```python
from build123d import *

# Parameters (mm, degrees)
SKETCH2_R                       = 11.10996
BOSS_EXTRUDE1_DEPTH             = 4.7625
SKETCH3_W                       = 3.175
SKETCH3_H                       = 181.991160274
CUT_EXTRUDE1_DEPTH              = 0.396875
FILLET1_R                       = 0.79375
F_9_64_0_14063_DIAMETER_HOLE1_D = 3.572002


with BuildPart() as part:
    # Sketch2 → Boss-Extrude1 (new body)
    with BuildSketch(Plane(origin=(0, 0, 0), x_dir=(0, 0, -1), z_dir=(1, 0, 0))):
        with BuildLine():
            Line((81.02619141, 88.258519733), (35.921024484, 114.3))
            ThreePointArc((35.921024484, 114.3), (0, 63.5), (-35.921024484, 114.3))
            Line((-35.921024484, 114.3), (-81.02619141, 88.258519733))
            ThreePointArc((-81.02619141, 88.258519733), (-54.99261314, 31.75), (-116.947215895, 26.041480267))
            Line((-116.947215895, 26.041480267), (-116.947215895, -26.041480267))
            ThreePointArc((-116.947215895, -26.041480267), (-54.99261314, -31.75), (-81.02619141, -88.258519733))
            Line((-81.02619141, -88.258519733), (-35.921024484, -114.3))
            ThreePointArc((-35.921024484, -114.3), (0, -63.5), (35.921024484, -114.3))
            Line((35.921024484, -114.3), (81.02619141, -88.258519733))
            ThreePointArc((81.02619141, -88.258519733), (54.99261314, -31.75), (116.947215895, -26.041480267))
            Line((116.947215895, -26.041480267), (116.947215895, 26.041480267))
            ThreePointArc((116.947215895, 26.041480267), (54.99261314, 31.75), (81.02619141, 88.258519733))
        make_face()
        with Locations(Location((0, 0, 0), (0, 0, 180))):
            Circle(SKETCH2_R, mode=Mode.SUBTRACT)
    extrude(amount=BOSS_EXTRUDE1_DEPTH)

    # Sketch3 → Cut-Extrude1 (cut)
    with BuildSketch(Plane.ZY):
        with Locations((0, 101.6)):
            Rectangle(SKETCH3_W, SKETCH3_H)
        Polygon((167.586415056, 94.92297474), (165.998915056, 97.672605397), (8.389946993, 6.67702526), (9.977446993, 3.927394603), align=None)
        Polygon((165.998915056, -97.672605397), (167.586415056, -94.92297474), (9.977446993, -3.927394603), (8.389946993, -6.67702526), align=None)
        with Locations((0, -101.6)):
            Rectangle(SKETCH3_W, SKETCH3_H)
        Polygon((-167.586415056, -94.92297474), (-165.998915056, -97.672605397), (-8.389946993, -6.67702526), (-9.977446993, -3.927394603), align=None)
        Polygon((-165.998915056, 97.672605397), (-167.586415056, 94.92297474), (-9.977446993, 3.927394603), (-8.389946993, 6.67702526), align=None)
    extrude(amount=-CUT_EXTRUDE1_DEPTH, mode=Mode.SUBTRACT)

    # Fillet1
    fillet1_edges = [part.edges().sort_by_distance(p)[0] for p in [
        (2.38125, 88.258519733, 81.02619141),
        (2.38125, 114.3, 35.921024484),
        (2.38125, 114.3, -35.921024484),
        (2.38125, 88.258519733, -81.02619141),
        (2.38125, 26.041480267, -116.947215895),
        (2.38125, -26.041480267, -116.947215895),
        (2.38125, -88.258519733, -81.02619141),
        (2.38125, -114.3, -35.921024484),
        (2.38125, -114.3, 35.921024484),
        (2.38125, -88.258519733, 81.02619141),
        (2.38125, -26.041480267, 116.947215895),
        (2.38125, 26.041480267, 116.947215895),
    ]]
    fillet(fillet1_edges, radius=FILLET1_R)

    # 9/64 (0.14063) Diameter Hole1 (through all)
    with Locations(Plane.ZY):
        with Locations((0, 25.4), (21.997045256, -12.7), (-21.997045256, -12.7)):
            Hole(F_9_64_0_14063_DIAMETER_HOLE1_D / 2)


solid = part.part
```
Part model, mm, in its own coordinate system. A direction names the side the tool comes from. Round coordinates to 2 decimals unless told otherwise and drop trailing zeros. Write each loop counter-clockwise with the first axis right and the second up, starting at its lowest first coordinate (ties: lowest second). Pieces come first, ordered by that corner, then holes. Notation, with made-up numbers: M 18,69.25 L 27,69.25 A29 cw 27,92.25 Z; hole C 6.25,5.5 d11. An arc over 180 degrees is marked long. One line per question, with ' | ' between items.
(1) Two-plate mould, pull along Z, no slides. Class faces 3 (the face through (2.348, 101.111, -58.764)), 4 (the face through (0, -59, -31)), 5 (the face through (0.196, 17.074, 32.747)): released by +Z, released by -Z, zero draft, split by the parting line, or undercut.
Answer key:
face 3: released by -Z | face 4: zero draft | face 5: undercut
(2) 3-axis set-ups, long thin cutter, end or side, ignore diameter. For faces 1 (the face through (0.2, -20.93, -39.43)), 2 (the face through (2.35, -32.61, -54.51)): which of +Z, -Z, +X, -X, +Y, -Y reach the whole face in a straight line?
Answer key:
face 1: -X | face 2: +X, -X
(3) Saw through at D-D on x = 1.55. Write the cut outline in (y, z) (1 decimal), then the cut area to 3 significant figures.
Answer key:
outline: M -113.3,-37.7 L -89.3,-79.2 A0.8 ccw -87.8,-79 A38.1 cw long -24.5,-115.6 A0.8 ccw -24,-116.9 L 24,-116.9 A0.8 ccw 24.5,-115.6 A38.1 cw long 87.8,-79 A0.8 ccw 89.3,-79.2 L 113.3,-37.7 A0.8 ccw 112.4,-36.6 A38.1 cw long 112.4,36.6 A0.8 ccw 113.3,37.7 L 89.3,79.2 A0.8 ccw 87.8,79 A38.1 cw long 24.5,115.6 A0.8 ccw 24,116.9 L -24,116.9 A0.8 ccw -24.5,115.6 A38.1 cw long -87.8,79 A0.8 ccw -89.3,79.2 L -113.3,37.7 A0.8 ccw -112.4,36.6 A38.1 cw long -112.4,-36.6 A0.8 ccw Z; hole C -12.7,-22 d3.6; hole C -12.7,22 d3.6; hole C 0,0 d22.2; hole C 25.4,0 d3.6 | area: 23,100 mm^2
(4) Saw through at A-A on y = 0. Write the cut outline in (x, z), then the cut area to 3 significant figures.
Answer key:
outline: M 0,-116.95 L 4.76,-116.95 L 4.76,-11.11 L 0,-11.11 Z; M 0,11.11 L 4.76,11.11 L 4.76,116.95 L 0,116.95 Z | area: 1,010 mm^2
(5) Pin check, flat tips, straight feed: pin 1 (1 mm diameter, centred on x = 3.5, z = 14.5, fed in from +Y); pin 2 (1 mm diameter, centred on x = 2.5, y = -57, fed in from +Z); pin 3 (2 mm diameter, centred on x = 2, z = -39, fed in from -Y). Stop position of each tip, or through.
Answer key:
pin 1: stops at y = 66.58 | pin 2: stops at z = 50.48 | pin 3: stops at y = -113.1
(6) Saw through at B-B on y = -50.8. Write the cut outline in (x, z), then the cut area to 3 significant figures.
Answer key:
outline: M 0,-49.89 L 4.76,-49.89 L 4.76,49.89 L 0,49.89 L 0,1.59 L 0.4,1.59 L 0.4,-1.59 L 0,-1.59 Z | area: 474 mm^2
(7) Probe line 1 along Y through (x, z) = (2.95, 0); line 2 along Z through (x, y) = (1.45, 24.5); line 3 along Y through (x, z) = (1.9, 89.5). List the from-to ranges inside material, lowest first.
Answer key:
line 1: y = -63.5 to -11.11, 11.11 to 23.61, 27.19 to 63.5 | line 2: z = -116.75 to -115.55, -60.42 to -1.54, 1.54 to 60.42, 115.55 to 116.75 | line 3: y = -12.73 to 12.73
(8) Saw through at C-C on z = -71.5. Write the cut outline in (x, y).
Answer key:
outline: M 0,-93.76 L 4.76,-93.76 L 4.76,-85.15 L 0,-85.15 Z; M 0,-16.45 L 4.76,-16.45 L 4.76,16.45 L 0,16.45 Z; M 0,85.15 L 4.76,85.15 L 4.76,93.76 L 0,93.76 Z
